from build123d import *

# Parameters (mm, degrees)
BOSS_EXTRUDE1_DEPTH = 6.35
CUT_EXTRUDE1_REACH  = 310.984
SKETCH3_R           = 15.875


with BuildPart() as part:
    # Sketch2 → Boss-Extrude1 (new body)
    with BuildSketch(Plane.XY):
        with BuildLine():
            Line((218.563766336, -180.975), (218.563766336, -104.775))
            ThreePointArc((218.563766336, -104.775), (207.627719332, -78.373047004), (181.225766336, -67.437))
            Line((181.225766336, -67.437), (-181.225766336, -67.437))
            ThreePointArc((-181.225766336, -67.437), (-207.627719332, -78.373047004), (-218.563766336, -104.775))
            Line((-218.563766336, -104.775), (-218.563766336, -180.975))
            ThreePointArc((-218.563766336, -180.975), (-207.627719332, -207.376952996), (-181.225766336, -218.313))
            Line((-181.225766336, -218.313), (181.225766336, -218.313))
            ThreePointArc((181.225766336, -218.313), (207.627719332, -207.376952996), (218.563766336, -180.975))
        make_face()
    extrude(amount=BOSS_EXTRUDE1_DEPTH)

    # Sketch3 → Cut-Extrude1 (cut, up to next)
    with BuildSketch(Plane.XY.offset(6.35), mode=Mode.PRIVATE) as cut_extrude1_sk1:
        with Locations((-38.1, -142.875)):
            Circle(SKETCH3_R)
    cut_extrude1_tool1 = extrude(cut_extrude1_sk1.sketch, amount=-CUT_EXTRUDE1_REACH, mode=Mode.PRIVATE) & part.part
    # Sketch3 → Cut-Extrude1 (cut, up to next)
    with BuildSketch(Plane.XY.offset(6.35), mode=Mode.PRIVATE) as cut_extrude1_sk2:
        with Locations((38.1, -142.875)):
            Circle(SKETCH3_R)
    cut_extrude1_tool2 = extrude(cut_extrude1_sk2.sketch, amount=-CUT_EXTRUDE1_REACH, mode=Mode.PRIVATE) & part.part
    add(cut_extrude1_tool1.solids().sort_by_distance((-38.1, -142.875, 6.35))[0], mode=Mode.SUBTRACT)
    add(cut_extrude1_tool2.solids().sort_by_distance((38.1, -142.875, 6.35))[0], mode=Mode.SUBTRACT)


solid = part.part
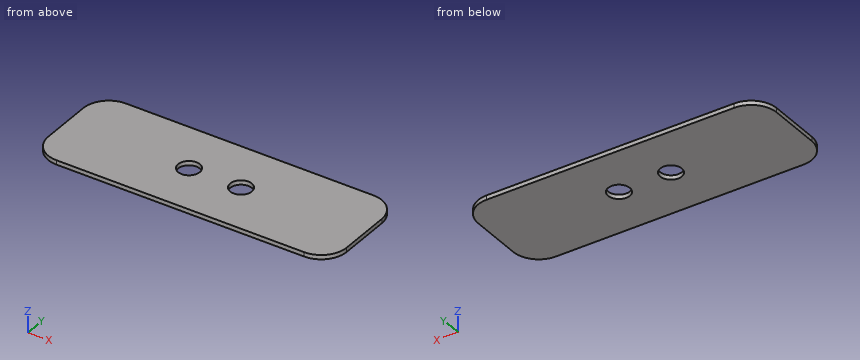
Design review of the part built by this model. Coordinates are the model's own, in mm. Round coordinates to 2 decimals unless told otherwise and drop trailing zeros. Order: outer loops, then holes, each group sorted by start corner. A loop starts at its lowest first (then second) coordinate and runs counter-clockwise, first axis right, second up.
1) For L1, parallel to Y at x = 39, z = 2.75; L2, parallel to X at y = -135, z = 3; L3, parallel to X at y = -155, z = 0.5, list the stretches that pass through material, from the lowest coordinate up.
The answers:
L1: y = -218.31 to -158.72, -127.03 to -67.44
L2: x = -218.56 to -51.88, -24.32 to 24.32, 51.88 to 218.56
L3: x = -218.56 to -48.35, -27.85 to 27.85, 48.35 to 218.56
2) Consider section C-C (y = -197). State the section outline as (x, z) points.
The answers:
outline: (-214.95, 0) - (214.95, 0) - (214.95, 6.35) - (-214.95, 6.35) - close
3) Consider section B-B (z = 2.25). State the section outline as (x, y) points (3 decimals), plus the area to 3 significant figures.
The answers:
outline: (-218.564, -180.975) arc R37.338 ccw to (-181.226, -218.313) - (181.226, -218.313) arc R37.338 ccw to (218.564, -180.975) - (218.564, -104.775) arc R37.338 ccw to (181.226, -67.437) - (-181.226, -67.437) arc R37.338 ccw to (-218.564, -104.775) - close; hole circle Ø31.75 at (-38.1, -142.875); hole circle Ø31.75 at (38.1, -142.875)
area: 63,200 mm2
4) Clearance check with a flat-ended pin moving along its axis: pin 1 Ø1 at (y, z) = (-96, 5.5) entering from +X. State where the tip first meets the part, or that it passes through.
The answers:
pin 1: stops at x = 217.64
5) Consider section A-A (x = -39). State the section outline as (y, z) points.
The answers:
outline: (-218.31, 0) - (-158.72, 0) - (-158.72, 6.35) - (-218.31, 6.35) - close; (-127.03, 0) - (-67.44, 0) - (-67.44, 6.35) - (-127.03, 6.35) - close
